from build123d import *

# Parameters (mm, degrees)
SKETCH_1_R             = 0.25
EXTRUDE_1_DEPTH        = 0.4
FILLET_1_R             = 0.5
FILLET_1_OF_MIRROR_1_R = 0.5


with BuildPart() as part:
    # Эскиз1 → Бобышка-Вытянуть1 (new body, symmetric)
    with BuildSketch(Plane.XY):
        with BuildLine():
            Line((2, 6.977225575), (0.5, 6.977225575))
            Line((0.5, 6.977225575), (0.5, 5.980740698))
            ThreePointArc((0.5, 5.980740698), (1.258735944, 5.876957254), (2, 5.684658438))
            Line((2, 5.684658438), (2, 6.977225575))
        make_face()
        with Locations((1.25, 6.427950493)):
            Circle(SKETCH_1_R, mode=Mode.SUBTRACT)
        with BuildLine():
            ThreePointArc((2, 5.684658438), (1.258735944, 5.876957254), (0.5, 5.980740698))
            Line((0.5, 5.980740698), (0.5, 5.477225575))
            ThreePointArc((0.5, 5.477225575), (5.494303444, -0.250259203), (0, -5.5))
            Line((0, -5.5), (0, -7))
            ThreePointArc((0, -7), (6.420680643, -1.51235373), (2, 5.684658438))
        make_face()
    extrude_1 = extrude(amount=EXTRUDE_1_DEPTH, both=True)

    # Скругление1
    fillet_1_edges = [part.edges().sort_by_distance(p)[0] for p in [
        (2, 6.977225575, 0),
        (2, 5.684658438, 0),
    ]]
    fillet(fillet_1_edges, radius=FILLET_1_R)

    # Зеркальное отражение1: Бобышка-Вытянуть1 across plane
    add(extrude_1.mirror(Plane(origin=(0, 0, 0.4), x_dir=(0, 0, 1), z_dir=(1, 0, 0))))

    # Скругление1 of Зеркальное отражение1
    fillet_1_of_mirror_1_edges = [part.edges().sort_by_distance(p)[0] for p in [
        (-2, 6.977225575, 0),
        (-2, 5.684658438, 0),
    ]]
    fillet(fillet_1_of_mirror_1_edges, radius=FILLET_1_OF_MIRROR_1_R)


solid = part.part
Can you work these out from the model? Positions are in its coordinate system, mm. Round coordinates to 2 decimals unless told otherwise and drop trailing zeros. Write each loop counter-clockwise with the first axis right and the second up, starting at its lowest first coordinate (ties: lowest second). Pieces come first, ordered by that corner, then holes. Notation, with made-up numbers: M 60.25,-40 L 95.25,-40 A25 ccw 95.25,-25 Z; hole C 40.5,67.5 d1. An arc over 180 degrees is marked long. Use a Markdown table: item, result.
Item 1: For pin 1 Ø5 at (x, y) = (3, -2.5) entering from -Z; pin 2 Ø1.5 at (x, y) = (-3.5, -0.5) entering from -Z, each with a flat end and sliding along its axis, tell me the tip position at first contact or that it passes through.
Found:
| item | result |
|---|---|
| pin 1 | stops at z = -0.4 |
| pin 2 | passes through |
Item 2: I want a section at D-D (z = -0.15). List the corners of the cut face in (x, y) for me.
Found:
| item | result |
|---|---|
| outline | M -2.32,5.57 A6.5 ccw long 2.32,5.57 A0.5 cw 2,6.04 L 2,6.48 A0.5 ccw 1.5,6.98 L 0.5,6.98 L 0.5,5.48 A5.5 cw long -0.5,5.48 L -0.5,6.98 L -1.5,6.98 A0.5 ccw -2,6.48 L -2,6.04 A0.5 cw Z; hole C -1.25,6.43 d0.5; hole C 1.25,6.43 d0.5 |
Item 3: If I drill on line 1 along Y through (x, z) = (-1.25, -0.1); line 2 along X through (y, z) = (-0.5, 0.25); line 3 along X through (y, z) = (1.5, 0.05), over which ranges is the centre line in solid material (lowest first)? Write a range as [from, to].
Found:
| item | result |
|---|---|
| line 1 | y = [-6.88, -5.36], [5.36, 6.18], [6.68, 6.98] |
| line 2 | x = [-6.5, -5.48], [5.48, 6.5] |
| line 3 | x = [-6.18, -5.29], [5.29, 6.18] |
Item 4: I want a section at A-A (y = -3.5). List the corners of the cut face in (x, z) for me.
Found:
| item | result |
|---|---|
| outline | M -5.77,-0.4 L -4.24,-0.4 L -4.24,0.4 L -5.77,0.4 Z; M 4.24,-0.4 L 5.77,-0.4 L 5.77,0.4 L 4.24,0.4 Z |
Item 5: I want a section at B-B (x = -1.25). List the corners of the cut face in (y, z) for me.
Found:
| item | result |
|---|---|
| outline | M -6.88,-0.4 L -5.36,-0.4 L -5.36,0.4 L -6.88,0.4 Z; M 5.36,-0.4 L 6.18,-0.4 L 6.18,0.4 L 5.36,0.4 Z; M 6.68,-0.4 L 6.98,-0.4 L 6.98,0.4 L 6.68,0.4 Z |
Item 6: I want a section at C-C (x = -5). List the corners of the cut face in (y, z) for me, and give its area (3 significant figures).
Found:
| item | result |
|---|---|
| outline | M -4.65,-0.4 L -2.29,-0.4 L -2.29,0.4 L -4.65,0.4 Z; M 2.29,-0.4 L 3.65,-0.4 L 3.65,0.4 L 2.29,0.4 Z |
| area | 2.98 mm2 |
